from build123d import *

# Parameters (mm, degrees)
SKETCH2_W           = 52.5507204
SKETCH2_H           = 51.48598542
SKETCH2_W_2         = 3.81
SKETCH2_H_2         = 2.54
BOSS_EXTRUDE1_DEPTH = 5.08
SKETCH3_W           = 47.4707204
SKETCH3_H           = 46.40598542
CUT_EXTRUDE1_DEPTH  = 3.81
SKETCH4_R           = 1.1303
CUT_EXTRUDE2_DEPTH  = 3.302
SKETCH5_R           = 5.08
CUT_EXTRUDE3_DEPTH  = 1.9304
SKETCH6_R           = 6.985
BOSS_EXTRUDE2_DEPTH = 38.1
SKETCH8_R           = 5.08
CUT_EXTRUDE4_DEPTH  = 38.1
SKETCH7_W           = 38.1
SKETCH7_H           = 20.32
BOSS_EXTRUDE3_DEPTH = 6.35
FILLET3_R           = 2.54


with BuildPart() as part:
    # Sketch2 → Boss-Extrude1 (new body)
    with BuildSketch(Plane(origin=(0, 0, 0), x_dir=(1, 0, 0), z_dir=(0, 1, 0))):
        with Locations((0, 3.81e-06)):
            Rectangle(SKETCH2_W, SKETCH2_H)
        with Locations((28.1803602, 1.27)):
            Rectangle(SKETCH2_W_2, SKETCH2_H_2)
        with Locations((-28.1803602, 1.2700127)):
            Rectangle(SKETCH2_W_2, SKETCH2_H_2)
    extrude(amount=BOSS_EXTRUDE1_DEPTH)

    # Sketch3 → Cut-Extrude1 (cut)
    with BuildSketch(Plane.XZ):
        with Locations((0, -3.81e-06)):
            Rectangle(SKETCH3_W, SKETCH3_H)
    extrude(amount=-CUT_EXTRUDE1_DEPTH, mode=Mode.SUBTRACT)

    # Sketch4 → Cut-Extrude2 (cut)
    with BuildSketch(Plane.XY):
        with Locations((28.1803602, 2.54)):
            Circle(SKETCH4_R)
        with Locations((-28.1803602, 2.54)):
            Circle(SKETCH4_R)
    extrude(amount=-CUT_EXTRUDE2_DEPTH, mode=Mode.SUBTRACT)

    # Sketch5 → Cut-Extrude3 (cut)
    with BuildSketch(Plane(origin=(0, 5.08, 0), x_dir=(1, 0, 0), z_dir=(0, 1, 0))):
        Circle(SKETCH5_R)
    extrude(amount=-CUT_EXTRUDE3_DEPTH, mode=Mode.SUBTRACT)

    # Sketch6 → Boss-Extrude2 (add)
    with BuildSketch(Plane(origin=(0, 5.08, 0), x_dir=(1, 0, 0), z_dir=(0, 1, 0))):
        Circle(SKETCH6_R)
    extrude(amount=BOSS_EXTRUDE2_DEPTH)

    # Sketch8 → Cut-Extrude4 (cut)
    with BuildSketch(Plane(origin=(0, 43.18, 0), x_dir=(1, 0, 0), z_dir=(0, 1, 0))):
        Circle(SKETCH8_R)
    extrude(amount=-CUT_EXTRUDE4_DEPTH, mode=Mode.SUBTRACT)

    # Sketch7 → Boss-Extrude3 (add)
    with BuildSketch(Plane(origin=(0, 43.18, 0), x_dir=(1, 0, 0), z_dir=(0, 1, 0))):
        Rectangle(SKETCH7_W, SKETCH7_H)
    extrude(amount=BOSS_EXTRUDE3_DEPTH)

    # Fillet3
    fillet3_edges = [part.edges().sort_by_distance(p)[0] for p in [
        (-19.05, 43.18, 0),
        (0, 43.18, 10.16),
        (19.05, 43.18, 0),
        (0, 43.18, -10.16),
    ]]
    fillet(fillet3_edges, radius=FILLET3_R)


solid = part.part
The listing builds one solid part. Answer for the finished solid, in the listing's coordinates (mm). A direction names the side the tool comes from. Coordinates: 2 decimals unless noted, no trailing zeros. Order: outer loops, then holes, each group sorted by start corner. A loop starts at its lowest first (then second) coordinate and runs counter-clockwise, first axis right, second up. Notation, with made-up numbers: (-16.75, 51) -> (-9.75, 51) arc R14 cw to (-9.75, 76) -> close; hole circle Ø2 at (-31, 22). An arc over 180 degrees is marked (long way). Answer in a Markdown table with one row per item. Add a question column.
Item 1: Determine the mould class of faces 4 (the face through (-18.326, 43.944, -0.142)), 5 (the face through (28, 1, -2.54)), 6 (the face through (-2, 0, 25)) for opening direction Y: +Y half, -Y half, draft (parallel to the pull), parting line (faces both ways), or undercut.
Item 2: Find section C-C (z = -14.5). Write down the section's boundary in (x, y), then the cut area to 3 significant figures.
Item 3: Find the intervals of material crossed by L1, parallel to Z at x = 0, y = 20 (3 decimals); L2, parallel to Y at x = -5, z = -5; L3, parallel to Y at x = 22, z = 16.5, in increasing order. Write a range as from..to.
Item 4: Find section B-B (x = -8.5). Write down the section's boundary in (y, z), then the cut area to 3 significant figures.
Item 5: Find section D-D (x = 0). Write down the section's boundary in (y, z) (3 decimals), then the cut area to 3 significant figures.
Item 6: Which of the six approach directions +Z, -Z, +X, -X, +Y, -Y give full straight-line access (tool end or side, diameter ignored) to faces 1 (the face through (28, 1, 0)), 2 (the face through (19.05, 48, 0)), 3 (the face through (26.275, 3, -14))?
Item 7: Find section A-A (y = 2.54). Write down the section's boundary in (x, z), then the cut area to 3 significant figures.
Item 8: Each of these flat-tipped pins is pushed along its axis until it touches: P1, Ø4, axis at x = 9.5, y = 47.5, coming from the -Z side; P2, Ø1.9, axis at x = 28.5, y = 2, coming from the -Z side; P3, Ø3, axis at x = -4, y = 47.5, coming from the +Z side. Where does it stop, or does it pass through?
Result set:
| question | item | result |
|---|---|---|
| 1 | face 4 | undercut |
| 1 | face 5 | draft |
| 1 | face 6 | -Y half |
| 2 | outline | (-26.28, 0) -> (-23.74, 0) -> (-23.74, 3.81) -> (23.74, 3.81) -> (23.74, 0) -> (26.28, 0) -> (26.28, 5.08) -> (-26.28, 5.08) -> close |
| 2 | area | 86.1 mm² |
| 3 | L1 | z = -6.985..-5.08, 5.08..6.985 |
| 3 | L2 | y = 3.81..5.08, 43.18..49.53 |
| 3 | L3 | y = 3.81..5.08 |
| 4 | outline | (0, -25.74) -> (5.08, -25.74) -> (5.08, 25.74) -> (0, 25.74) -> (0, 23.2) -> (3.81, 23.2) -> (3.81, -23.2) -> (0, -23.2) -> close; (43.18, -7.62) arc R2.54 ccw to (45.72, -10.16) -> (49.53, -10.16) -> (49.53, 10.16) -> (45.72, 10.16) arc R2.54 ccw to (43.18, 7.62) -> close |
| 4 | area | 211 mm² |
| 5 | outline | (0, -25.743) -> (5.08, -25.743) -> (5.08, -6.985) -> (43.18, -6.985) -> (43.18, -7.62) arc R2.54 ccw to (45.72, -10.16) -> (49.53, -10.16) -> (49.53, 10.16) -> (45.72, 10.16) arc R2.54 ccw to (43.18, 7.62) -> (43.18, 6.985) -> (5.08, 6.985) -> (5.08, 25.743) -> (0, 25.743) -> (0, 23.203) -> (3.81, 23.203) -> (3.81, 5.08) -> (43.18, 5.08) -> (43.18, -5.08) -> (3.81, -5.08) -> (3.81, -23.203) -> (0, -23.203) -> close |
| 5 | area | 343 mm² |
| 6 | face 1 | +Z, +X, +Y, -Y |
| 6 | face 2 | +Z, -Z, +X, +Y |
| 6 | face 3 | -Z, +X, +Y, -Y |
| 7 | outline | (-30.09, -2.54) -> (-29.31, -2.54) -> (-29.31, 0) -> (-30.09, 0) -> close; (-27.05, -2.54) -> (-26.28, -2.54) -> (-26.28, -25.74) -> (26.28, -25.74) -> (26.28, -2.54) -> (27.05, -2.54) -> (27.05, 0) -> (26.28, 0) -> (26.28, 25.74) -> (-26.28, 25.74) -> (-26.28, 0) -> (-27.05, 0) -> close; (29.31, -2.54) -> (30.09, -2.54) -> (30.09, 0) -> (29.31, 0) -> close; hole (-23.74, -23.2) -> (23.74, -23.2) -> (23.74, 23.2) -> (-23.74, 23.2) -> close |
| 7 | area | 511 mm² |
| 8 | P1 | stops at z = -10.16 |
| 8 | P2 | stops at z = -2.54 |
| 8 | P3 | stops at z = 10.16 |
